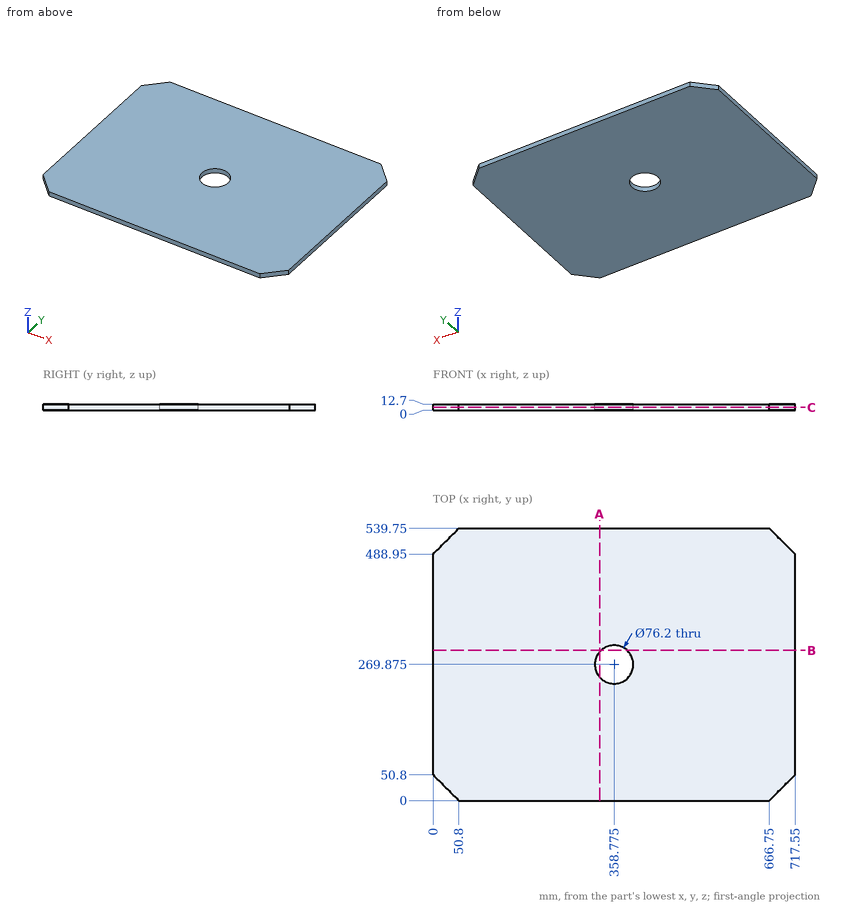
For this review, use the dimensioned drawing (mm, ordinates from the lowest corner) and the shaded views. Coordinates: 2 decimals unless noted, no trailing zeros. Write each loop counter-clockwise with the first axis right and the second up, starting at its lowest first coordinate (ties: lowest second). Pieces come first, ordered by that corner, then holes. Notation, with made-up numbers: (3.5, 28) - (54.5, 28) arc R25 ccw to (54.5, 55) - close; hole circle Ø8 at (19, -4.5). An arc over 180 degrees is marked (long way). Answer in a Markdown table with one row per item. Add a question column.
Q1. Consider section B-B on y = 298. Give the boundary of the cut face in (x, z).
Q2. To check wall thickness, follow line 1 along X through (y, z) = (297, 0.5); line 2 along Y through (x, z) = (46, 9.25); line 3 along Y through (x, z) = (391, 5). State the ranges of each line that lie inside material, in increasing order. Write a range as from..to.
Q3. Consider section C-C on z = 6. Give the boundary of the cut face in (x, y) (3 decimals).
Q4. Consider section A-A on x = 330. Give the boundary of the cut face in (y, z), then the cut area to 3 significant figures.
Answers below:
| question | item | result |
|---|---|---|
| 1 | outline | (0, 0) - (333.07, 0) - (333.07, 12.7) - (0, 12.7) - close; (384.48, 0) - (717.55, 0) - (717.55, 12.7) - (384.48, 12.7) - close |
| 2 | line 1 | 0..332.02, 385.53..717.55 |
| 2 | line 2 | 4.8..534.95 |
| 2 | line 3 | 0..249.55, 290.2..539.75 |
| 3 | outline | (0, 50.8) - (50.8, 0) - (666.75, 0) - (717.55, 50.8) - (717.55, 488.95) - (666.75, 539.75) - (50.8, 539.75) - (0, 488.95) - close; hole circle Ø76.2 at (358.775, 269.875) |
| 4 | outline | (0, 0) - (244.9, 0) - (244.9, 12.7) - (0, 12.7) - close; (294.85, 0) - (539.75, 0) - (539.75, 12.7) - (294.85, 12.7) - close |
| 4 | area | 6,220 mm² |
